Part model, mm, in its own coordinate system. A direction names the side the tool comes from. Coordinates: 2 decimals unless noted, no trailing zeros. Loops run counter-clockwise (first coordinate to the right, second up) from the corner with the lowest first, then second, coordinate; pieces in that order, holes last. Notation, with made-up numbers: (5.5, 20) -> (57.5, 20) arc R5 cw to (57.5, 27) -> close; hole circle Ø11 at (-37.5, 71.5). An arc over 180 degrees is marked (long way). One line per question, with ' | ' between items. Start each with the question number.
1) Cut at C-C (z = 2.5). List the corners of the cut face in (x, y), plus the area to 3 significant figures.
2) Cut at D-D (x = -2.5). List the corners of the cut face in (y, z).
3) Probe L1, parallel to Z at x = 3, y = 0.3; L2, parallel to Y at x = -3.5, z = -8.25; L3, parallel to Z at x = -0.5, y = 3.9. List the from-to ranges inside material, lowest first. Write a range as from..to.
4) Drop flat-ended pins along their axis: pin 1 (3 mm diameter, centred on x = 3, z = -10, fed in from +Y); pin 2 (0.6 mm diameter, centred on y = 0.5, z = -12, fed in from +X); pin 3 (1.5 mm diameter, centred on x = -0.5, y = 2.5, fed in from -Z). Give the stop position or say it passes through.
5) Cut at B-B (y = 1). List the corners of the cut face in (x, z), plus the area to 3 significant figures.
6) 3-axis set-ups, long thin cutter, end or side, ignore diameter. For faces 4 (the face through (2.5, 1.99, 3.6)), 5 (the face through (-4.572, 1, -14)), 6 (the face through (4.572, 1, -9)): which of +Z, -Z, +X, -X, +Y, -Y reach the whole face in a straight line?
7) Two-plate mould, pull along Z, no slides. Class faces 1 (the face through (4.372, 3.926, -7.145)), 2 (the face through (4, 1, -12.739)), 3 (the face through (4.572, 1, -14)): released by +Z, released by -Z, zero draft, split by the parting line, or undercut.
8) Cut at A-A (x = 0). List the corners of the cut face in (y, z), plus the area to 3 significant figures.
from build123d import *
from OCP.BRepFilletAPI import BRepFilletAPI_MakeChamfer

# Parameters (mm, degrees)
EXTRUDE1_DEPTH        = 4.826
EXTRUDE1_DEPTH_BACK   = 4.826
SKETCH10_R            = 1.8
SKETCH10_W            = 1.233836604
SKETCH10_H            = 1.6931216
EXTRUDE5_DEPTH        = 16.428369203
SKETCH6_W             = 0.8
SKETCH6_H             = 0.52
EXTRUDE6_DEPTH        = 13
EXTRUDE7_START        = -0.52
EXTRUDE7_DEPTH        = 0.52
CHAMFER1_SIZE         = 0.254
SKETCH12_W            = 7.379682426
SKETCH12_H            = 2.736118788
EXTRUDE8_DEPTH        = 0.254
SKETCH13_W            = 7.379682426
SKETCH13_H            = 2.736118788
EXTRUDE9_DEPTH        = 0.254
CHAMFER2_SIZE         = 0.508
CHAMFER2_SIZE2        = 0.91645626
CHAMFER3_SIZE         = 0.2032
CHAMFER3_SIZE2        = 0.366582504
CHAMFER3_SIZE2_2      = 0.605677555
CHAMFER3_SIZE2_3      = 0.557834937
EXTRUDE10_DEPTH       = 1.016
ESBO_O1_W             = 2.508369598
ESBO_O1_H             = 14.0227971
CORTE_EXTRUS_O1_DEPTH = 2.54
SKETCH17_W            = 14.984360746
SKETCH17_H            = 12.426120952
CUT_EXTRUDE1_DEPTH    = 22.464410101


with BuildPart() as part:
    # Sketch2 → Extrude1 (new, two sides)
    with BuildSketch(Plane(origin=(0, 0, 0), x_dir=(0, 0, -1), z_dir=(1, 0, 0))) as extrude1_sk:
        Polygon((14.3005, 0), (-1.0795, 0), (-1.0795, 4.5), (7.124012877, 4.5), (7.8005, 1.3), (14.3005, 1.3), align=None)
    extrude(amount=EXTRUDE1_DEPTH)
    extrude(extrude1_sk.sketch, amount=-EXTRUDE1_DEPTH_BACK)

    # Sketch10 → Extrude5 (cut, through all)
    with BuildSketch(Plane(origin=(0, 1.3, 0), x_dir=(1, 0, 0), z_dir=(0, 1, 0))):
        with Locations(Location((0, 11.3505, 0), (0, 0, 270))):
            Circle(SKETCH10_R)
        with Locations((-4.209081698, 11.892729701)):
            Rectangle(SKETCH10_W, SKETCH10_H)
        with Locations((4.209081698, 11.892729701)):
            Rectangle(SKETCH10_W, SKETCH10_H)
    extrude(amount=-EXTRUDE5_DEPTH, mode=Mode.SUBTRACT)

    # Sketch6 → Extrude6 (add)
    with BuildSketch(Plane.XY.offset(1.0795)):
        with Locations((2.54, 2.25)):
            Rectangle(SKETCH6_W, SKETCH6_H)
        with Locations((-2.54, 2.25)):
            Rectangle(SKETCH6_W, SKETCH6_H)
        with Locations((0, 2.25)):
            Rectangle(SKETCH6_W, SKETCH6_H)
    extrude(amount=EXTRUDE6_DEPTH)

    # Sketch11 → Extrude7 (add)
    with BuildSketch(Plane(origin=(0, 2.51, 0), x_dir=(1, 0, 0), z_dir=(0, 1, 0)).offset(EXTRUDE7_START)):
        Polygon((-2.94, -2.0475), (-3.29, -2.0475), (-3.29, -3.5395), (-3.2004, -3.5395), (-3.2004, -3.7747), (-2.94, -4.0795), align=None)
        Polygon((-1.79, -2.0475), (-2.14, -2.0475), (-2.14, -4.0795), (-1.8796, -3.7747), (-1.8796, -3.5395), (-1.79, -3.5395), align=None)
        Polygon((-0.4, -2.0475), (-0.75, -2.0475), (-0.75, -3.5395), (-0.6604, -3.5395), (-0.6604, -3.7747), (-0.4, -4.0795), align=None)
        Polygon((0.75, -2.0475), (0.4, -2.0475), (0.4, -4.0795), (0.6604, -3.7747), (0.6604, -3.5395), (0.75, -3.5395), align=None)
        Polygon((2.14, -2.0475), (1.79, -2.0475), (1.79, -3.5395), (1.8796, -3.5395), (1.8796, -3.7747), (2.14, -4.0795), align=None)
        Polygon((3.29, -2.0475), (2.94, -2.0475), (2.94, -4.0795), (3.2004, -3.7747), (3.2004, -3.5395), (3.29, -3.5395), align=None)
    extrude(amount=EXTRUDE7_DEPTH)

    # Chamfer1
    chamfer1_edges = [part.edges().sort_by_distance(p)[0] for p in [
        (-2.14, 2.25, 14.0795),
        (-2.94, 2.25, 14.0795),
        (2.94, 2.25, 14.0795),
        (2.14, 2.25, 14.0795),
        (0.4, 2.25, 14.0795),
        (-0.4, 2.25, 14.0795),
    ]]
    chamfer(chamfer1_edges, length=CHAMFER1_SIZE)

    # Sketch12 → Extrude8 (cut)
    with BuildSketch(Plane.ZY.offset(4.826)):
        with Locations((-11.490341213, 1.368059394)):
            Rectangle(SKETCH12_W, SKETCH12_H)
    extrude(amount=-EXTRUDE8_DEPTH, mode=Mode.SUBTRACT)

    # Sketch13 → Extrude9 (cut)
    with BuildSketch(Plane(origin=(4.826, 0, 0), x_dir=(0, 0, -1), z_dir=(1, 0, 0))):
        with Locations((11.490341213, 1.368059394)):
            Rectangle(SKETCH13_W, SKETCH13_H)
    extrude(amount=-EXTRUDE9_DEPTH, mode=Mode.SUBTRACT)

    # Chamfer2: one chamfer whose edges measure the first distance from different faces: ONE call of the kernel's chamfer builder (chamfer() names one face for all edges)
    chamfer2_edges_1 = [part.edges().sort_by_distance(p)[0] for p in [
        (-4.826, 4.5, -3.022256439),
    ]]
    chamfer2_side_1 = [part.faces().sort_by_distance(p)[0] for p in [
        (-4.826, 2.217055195, -3.243165334),
    ]]
    chamfer2_edges_2 = [part.edges().sort_by_distance(p)[0] for p in [
        (4.826, 4.5, -3.022256439),
    ]]
    chamfer2_side_2 = [part.faces().sort_by_distance(p)[0] for p in [
        (4.826, 2.217055195, -3.243165334),
    ]]
    chamfer2 = BRepFilletAPI_MakeChamfer(part.part.solid().wrapped)
    for e in chamfer2_edges_1:
        chamfer2.Add(CHAMFER2_SIZE, CHAMFER2_SIZE2, e.wrapped, chamfer2_side_1[0].wrapped)  # the first distance lies on this face
    for e in chamfer2_edges_2:
        chamfer2.Add(CHAMFER2_SIZE, CHAMFER2_SIZE2, e.wrapped, chamfer2_side_2[0].wrapped)  # the first distance lies on this face
    add(Compound.cast(chamfer2.Shape()), mode=Mode.REPLACE)

    # Chamfer3: one chamfer whose edges measure the first distance from different faces: ONE call of the kernel's chamfer builder (chamfer() names one face for all edges)
    chamfer3_edges_1 = [part.edges().sort_by_distance(p)[0] for p in [
        (0, 4.5, 1.0795),
    ]]
    chamfer3_side_1 = [part.faces().sort_by_distance(p)[0] for p in [
        (0, 4.5, -3.022256439),
    ]]
    chamfer3_edges_2 = [part.edges().sort_by_distance(p)[0] for p in [
        (-4.36777187, 4.246, 1.0795),
    ]]
    chamfer3_side_2 = [part.faces().sort_by_distance(p)[0] for p in [
        (-4.368765147, 4.245449417, -3.049162718),
    ]]
    chamfer3_edges_3 = [part.edges().sort_by_distance(p)[0] for p in [
        (4.36777187, 4.246, 1.0795),
    ]]
    chamfer3_side_3 = [part.faces().sort_by_distance(p)[0] for p in [
        (4.368765147, 4.245449417, -3.049162718),
    ]]
    chamfer3_edges_4 = [part.edges().sort_by_distance(p)[0] for p in [
        (0, 4.5, -7.124012877),
    ]]
    chamfer3_side_4 = [part.faces().sort_by_distance(p)[0] for p in [
        (0, 4.5, -3.022256439),
    ]]
    chamfer3_edges_5 = [part.edges().sort_by_distance(p)[0] for p in [
        (-4.36777187, 4.246, -7.177709043),
    ]]
    chamfer3_side_5 = [part.faces().sort_by_distance(p)[0] for p in [
        (-4.368765147, 4.245449417, -3.049162718),
    ]]
    chamfer3_edges_6 = [part.edges().sort_by_distance(p)[0] for p in [
        (4.36777187, 4.246, -7.177709043),
    ]]
    chamfer3_side_6 = [part.faces().sort_by_distance(p)[0] for p in [
        (4.368765147, 4.245449417, -3.049162718),
    ]]
    chamfer3 = BRepFilletAPI_MakeChamfer(part.part.solid().wrapped)
    for e in chamfer3_edges_1:
        chamfer3.Add(CHAMFER3_SIZE, CHAMFER3_SIZE2, e.wrapped, chamfer3_side_1[0].wrapped)  # the first distance lies on this face
    for e in chamfer3_edges_2:
        chamfer3.Add(CHAMFER3_SIZE, CHAMFER3_SIZE2, e.wrapped, chamfer3_side_2[0].wrapped)  # the first distance lies on this face
    for e in chamfer3_edges_3:
        chamfer3.Add(CHAMFER3_SIZE, CHAMFER3_SIZE2, e.wrapped, chamfer3_side_3[0].wrapped)  # the first distance lies on this face
    for e in chamfer3_edges_4:
        chamfer3.Add(CHAMFER3_SIZE, CHAMFER3_SIZE2_2, e.wrapped, chamfer3_side_4[0].wrapped)  # the first distance lies on this face
    for e in chamfer3_edges_5:
        chamfer3.Add(CHAMFER3_SIZE, CHAMFER3_SIZE2_3, e.wrapped, chamfer3_side_5[0].wrapped)  # the first distance lies on this face
    for e in chamfer3_edges_6:
        chamfer3.Add(CHAMFER3_SIZE, CHAMFER3_SIZE2_3, e.wrapped, chamfer3_side_6[0].wrapped)  # the first distance lies on this face
    add(Compound.cast(chamfer3.Shape()), mode=Mode.REPLACE)

    # Sketch15 → Extrude10 (add)
    with BuildSketch(Plane.XY.offset(4.0795)):
        with BuildLine():
            Line((-2.14, 2.51), (-2.94, 2.51))
            ThreePointArc((-2.94, 2.51), (-3.017074418, 2.25), (-2.94, 1.99))
            Line((-2.94, 1.99), (-2.14, 1.99))
            ThreePointArc((-2.14, 1.99), (-2.062925582, 2.25), (-2.14, 2.51))
        make_face()
    extrude(amount=-EXTRUDE10_DEPTH)

    # Esboço1 → Corte-extrusão1 (cut)
    with BuildSketch(Plane(origin=(0, 2.51, 0), x_dir=(1, 0, 0), z_dir=(0, 1, 0))):
        with Locations((0.046451289, -8.09089855)):
            Rectangle(ESBO_O1_W, ESBO_O1_H)
    extrude(amount=-CORTE_EXTRUS_O1_DEPTH, mode=Mode.SUBTRACT)

    # Sketch17 → Cut-Extrude1 (cut, through all)
    with BuildSketch(Plane.XY.offset(6.1245)):
        Rectangle(SKETCH17_W, SKETCH17_H)
    extrude(amount=CUT_EXTRUDE1_DEPTH, mode=Mode.SUBTRACT)


solid = part.part
Reported:
1) outline: (-3.29, 1.99) -> (-1.79, 1.99) -> (-1.79, 2.51) -> (-3.29, 2.51) -> close; (1.79, 1.99) -> (3.29, 1.99) -> (3.29, 2.51) -> (1.79, 2.51) -> close | area: 1.56 mm²
2) outline: (0, -14.3) -> (1.3, -14.3) -> (1.3, -7.8) -> (3.91, -7.25) -> (4.5, -6.92) -> (4.5, 0.88) -> (4.13, 1.08) -> (2.51, 1.08) -> (2.51, 6.12) -> (1.99, 6.12) -> (1.99, 1.08) -> (0, 1.08) -> close
3) L1: z = -14.3..1.08 | L2: y = 0..1.3 | L3: z = -7.25..1.08
4) pin 1: stops at y = 1.3 | pin 2: stops at x = 3.59 | pin 3: stops at z = -7.71
5) outline: (-4.83, -7.8) -> (-4.57, -7.8) -> (-4.57, -11.05) -> (-3.59, -11.05) -> (-3.59, -12.74) -> (-4.57, -12.74) -> (-4.57, -14.3) -> (4.57, -14.3) -> (4.57, -12.74) -> (3.59, -12.74) -> (3.59, -11.05) -> (4.57, -11.05) -> (4.57, -7.8) -> (4.83, -7.8) -> (4.83, 1.08) -> (-4.83, 1.08) -> close; hole circle Ø3.6 at (0, -11.35) | area: 132 mm²
6) face 4: +Z, +X, -X, -Y | face 5: -Z, -X, +Y, -Y | face 6: -Z, +X, +Y, -Y
7) face 1: released by -Z | face 2: undercut | face 3: zero draft
8) outline: (0, -14.3) -> (1.3, -14.3) -> (1.3, -13.15) -> (0, -13.15) -> close; (0, -9.55) -> (1.3, -9.55) -> (1.3, -7.8) -> (3.91, -7.25) -> (4.5, -6.92) -> (4.5, 0.88) -> (4.13, 1.08) -> (0, 1.08) -> close | area: 42.6 mm²
